Work out the finished part from the listing and answer in its coordinate system (mm). Face numbers are marked on the shaded views. A direction names the side the tool comes from. Give positions to 0.01 mm unless a question says otherwise; leave off trailing zeros. Loops run counter-clockwise (first coordinate to the right, second up) from the corner with the lowest first, then second, coordinate; pieces in that order, holes last. Notation, with made-up numbers: M 23,41 L 79,41 A6 ccw 79,49 Z; hole C 16,-23.75 d5. An arc over 180 degrees is marked long. Use a Markdown table: item, result.
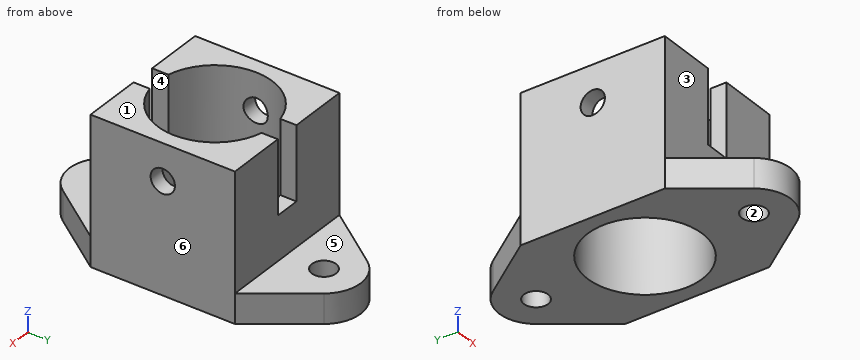
```python
from build123d import *

# Parameters (mm, degrees)
SKETCH_1_W          = 19.6
SKETCH_1_H          = 19.6
SKETCH_1_R          = 7.8
EXTRUDE_1_DEPTH     = 20
SKETCH_2_R          = 1.65
EXTRUDE_2_DEPTH     = 4
SKETCH_3_R          = 1.65
CUT_EXTRUDE_1_DEPTH = 35.295772334
SKETCH_4_W          = 3.5
SKETCH_4_H          = 19.6
CUT_EXTRUDE_2_DEPTH = 10


with BuildPart() as part:
    # 草图1 → 凸台-拉伸1 (new body)
    with BuildSketch(Plane.XY):
        Rectangle(SKETCH_1_W, SKETCH_1_H)
        Circle(SKETCH_1_R, mode=Mode.SUBTRACT)
    extrude(amount=EXTRUDE_1_DEPTH)

    # 草图2 → 凸台-拉伸2 (add)
    # profile 1 of 2: a face of its own
    with BuildSketch(Plane(origin=(0, 0, 0), x_dir=(-1, 0, 0), z_dir=(0, 0, -1))):
        with BuildLine():
            Line((-9.8, 9.8), (-4.048248513, 17.734567085))
            ThreePointArc((-4.048248513, 17.734567085), (0, 19.8), (4.048248513, 17.734567085))
            Line((4.048248513, 17.734567085), (9.8, 9.8))
            Line((9.8, 9.8), (-9.8, 9.8))
        make_face()
        with Locations((0, 14.8)):
            Circle(SKETCH_2_R, mode=Mode.SUBTRACT)
    # profile 2 of 2: a face of its own
    with BuildSketch(Plane(origin=(0, 0, 0), x_dir=(-1, 0, 0), z_dir=(0, 0, -1))):
        with BuildLine():
            Line((-9.8, -9.8), (9.8, -9.8))
            Line((9.8, -9.8), (4.048248513, -17.734567085))
            ThreePointArc((4.048248513, -17.734567085), (0, -19.8), (-4.048248513, -17.734567085))
            Line((-4.048248513, -17.734567085), (-9.8, -9.8))
        make_face()
        with Locations(Location((0, -14.8, 0), (0, 0, 180))):
            Circle(SKETCH_2_R, mode=Mode.SUBTRACT)
    extrude(amount=-EXTRUDE_2_DEPTH)

    # 草图3 → 切除-拉伸1 (cut, through all)
    with BuildSketch(Plane(origin=(9.8, 0, 0), x_dir=(0, 0, -1), z_dir=(1, 0, 0))):
        with Locations((-15, 0)):
            Circle(SKETCH_3_R)
    extrude(amount=-CUT_EXTRUDE_1_DEPTH, mode=Mode.SUBTRACT)

    # 草图4 → 切除-拉伸2 (cut)
    with BuildSketch(Plane.XY.offset(20)):
        Rectangle(SKETCH_4_W, SKETCH_4_H)
    extrude(amount=-CUT_EXTRUDE_2_DEPTH, mode=Mode.SUBTRACT)


solid = part.part
```
(1) A cutting plane is placed at B-B (y = 0). Write down the section's boundary in (x, z), and give its area (3 significant figures).
Entries:
| item | result |
|---|---|
| outline | M -9.8,0 L -7.8,0 L -7.8,13.35 L -9.8,13.35 Z; M -9.8,16.65 L -7.8,16.65 L -7.8,20 L -9.8,20 Z; M 7.8,0 L 9.8,0 L 9.8,13.35 L 7.8,13.35 Z; M 7.8,16.65 L 9.8,16.65 L 9.8,20 L 7.8,20 Z |
| area | 66.8 mm² |
(2) Consider probe 1 along Y at (x, z) = (0, 2.9); probe 2 along Y at (x, z) = (8.8, 15); probe 3 along Y at (x, z) = (0, 7). Determine where each line is inside the solid, lowest interval first. Write a range as [from, to].
Entries:
| item | result |
|---|---|
| probe 1 | y = [-19.8, -16.45], [-13.15, -7.8], [7.8, 13.15], [16.45, 19.8] |
| probe 2 | y = [-9.8, -1.65], [1.65, 9.8] |
| probe 3 | y = [-9.8, -7.8], [7.8, 9.8] |
(3) A cutting plane is placed at D-D (z = 18.75). Write down the section's boundary in (x, y), and give its area (3 significant figures).
Entries:
| item | result |
|---|---|
| outline | M -9.8,-9.8 L -1.75,-9.8 L -1.75,-7.6 A7.8 cw -1.75,7.6 L -1.75,9.8 L -9.8,9.8 Z; M 1.75,-9.8 L 9.8,-9.8 L 9.8,9.8 L 1.75,9.8 L 1.75,7.6 A7.8 cw 1.75,-7.6 Z |
| area | 179 mm² |
(4) Given P1, Ø4, axis at x = 0, z = 13, coming from the +Y side; P2, Ø0.7, axis at x = 0.5, y = 9, coming from the +Z side; P3, Ø1, axis at x = 2, y = 12.5, coming from the +Z side, each flat-ended and moving along its own axis, determine where each tip first touches the part or whether it passes through.
Entries:
| item | result |
|---|---|
| P1 | stops at y = 9.8 |
| P2 | stops at z = 10 |
| P3 | stops at z = 4 |
(5) A cutting plane is placed at A-A (z = 15). Write down the section's boundary in (x, y), and give its area (3 significant figures).
Entries:
| item | result |
|---|---|
| outline | M -9.8,-9.8 L -1.75,-9.8 L -1.75,-7.6 A7.8 cw -7.62,-1.65 L -9.8,-1.65 Z; M -9.8,1.65 L -7.62,1.65 A7.8 cw -1.75,7.6 L -1.75,9.8 L -9.8,9.8 Z; M 1.75,-9.8 L 9.8,-9.8 L 9.8,-1.65 L 7.62,-1.65 A7.8 cw 1.75,-7.6 Z; M 1.75,7.6 A7.8 cw 7.62,1.65 L 9.8,1.65 L 9.8,9.8 L 1.75,9.8 Z |
| area | 165 mm² |
(6) Which of the six approach directions +Z, -Z, +X, -X, +Y, -Y give full straight-line access (tool end or side, diameter ignored) to the marked faces 4, 5 and 6?
Entries:
| item | result |
|---|---|
| face 4 | +Z, +Y, -Y |
| face 5 | +Z, +X, -X, +Y |
| face 6 | +Z, -Z, +X, +Y, -Y |
(7) The mould has two halves that part along Y. Classify the marked faces 1, 2 and 3: released by +Y, released by -Y, zero draft, split by the parting line, or undercut.
Entries:
| item | result |
|---|---|
| face 1 | zero draft |
| face 2 | undercut |
| face 3 | released by -Y |
(8) A cutting plane is placed at C-C (x = 0). Write down the section's boundary in (y, z).
Entries:
| item | result |
|---|---|
| outline | M -19.8,0 L -16.45,0 L -16.45,4 L -19.8,4 Z; M -13.15,0 L -7.8,0 L -7.8,10 L -9.8,10 L -9.8,4 L -13.15,4 Z; M 7.8,0 L 13.15,0 L 13.15,4 L 9.8,4 L 9.8,10 L 7.8,10 Z; M 16.45,0 L 19.8,0 L 19.8,4 L 16.45,4 Z |
